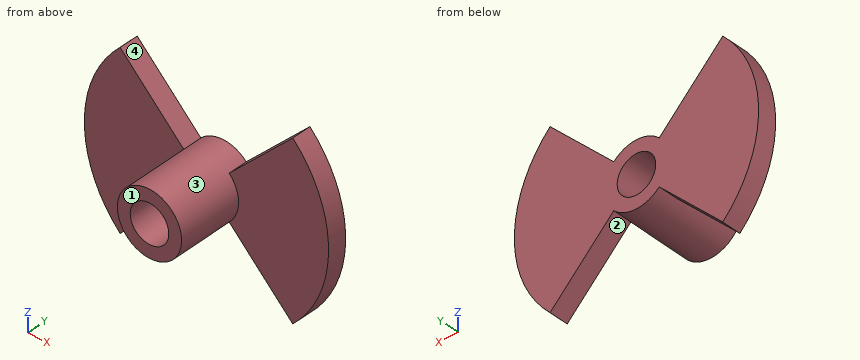
Autodesk Inventor part; units mm, degrees
ref_plane "YZ Plane" through (0, 0, 0) normal (1, 0, 0) x (0, 1, 0)
ref_plane "XZ Plane" through (0, 0, 0) normal (0, 1, 0) x (-1, 0, 0)
ref_plane "XY Plane" through (0, 0, 0) normal (0, 0, 1) x (1, 0, 0)
sketch "Sketch1" plane through (0, 0, 0) normal (0, 1, 0) x (-1, 0, 0)
  circle A0 centre (0, 0) radius 2.5
  circle A1 centre (0, 0) radius 1.5
  dimension "d1" = 3
  dimension "d2" = 1
extrude "Extrusion1" add sketch "Sketch1" along normal blind 5
sketch "Sketch2" plane through (0, 5, 0) normal (0, 1, 0) x (1, 0, 0)
  circle A0 centre (0, 0) radius 1.5
  circle A1 centre (0, 0) radius 9.5
  line L0 (-6.7175, -6.7175) -> (6.7175, 6.7175)
  line L1 (-6.7175, 6.7175) -> (6.7175, -6.7175)
  line L2 (-9.5, 0) -> (9.5, 0) construction
  circle A2 centre (0, 0) radius 2.5
  point P0 (1.7678, -1.7678)
  point P1 (1.7678, 1.7678)
  point P2 (-1.7678, 1.7678)
  point P3 (-1.7678, -1.7678)
  dimension "d5" = 19
  dimension "d6" = 45
  dimension "d7" = 45
extrude "Extrusion2" add sketch "Sketch2" along normal blind 1.5 contours A0 L0 A2 L1 | A0 L1 A2 L0 | L1 A2 L0 A0 | A0 L0 A2 L1 | L0 A1 L1 A2 | A2 L0 A1 L1 picked at (6.8013, -2.1485) picked at (-6.4568, -3.0059)
equation "\"d7\" = d6"
properties part number "Helice"
The listing builds one solid part. Answer for the finished solid, in the listing's coordinates (mm). Face numbers are marked on the shaded views. A direction names the side the tool comes from. Round coordinates to 2 decimals unless told otherwise and drop trailing zeros. Loops run counter-clockwise (first coordinate to the right, second up) from the corner with the lowest first, then second, coordinate; pieces in that order, holes last. Notation, with made-up numbers: (-38, 48) - (-23, 48) arc R6 ccw to (-23, 56) - close; hole circle Ø5 at (2.25, 20). An arc over 180 degrees is marked (long way). Return JSON: item names as keys, results as strings. Group by question number.
1. The part is cut by section C-C on z = -5.25. Determine the outline of the cut face in (x, y).
2. Which of the six approach directions +Z, -Z, +X, -X, +Y, -Y give full straight-line access (tool end or side, diameter ignored) to the marked faces 1, 2, 3 and 4?
3. The part is cut by section B-B on y = 5.75. Determine the outline of the cut face in (x, z).
4. The part is cut by section D-D on z = 2.75. Determine the outline of the cut face in (x, y), then the cut area to 3 significant figures.
5. Each of these flat-tipped pins is pushed along its axis until it touches: P1, Ø3, axis at x = -2.5, z = 5, coming from the +Y side; P2, Ø3, axis at x = 2, y = 3.5, coming from the -Z side; P3, Ø6, axis at x = -7, z = -0.5, coming from the -Y side. Where does it stop, or does it pass through?
6. The part is cut by section A-A on z = -2.25. Determine the outline of the cut face in (x, y).
7. Consider probe 1 along X at (y, z) = (3, 0); probe 2 along Y at (x, z) = (3.25, 2). Determine where each line is inside the solid, lowest interval first.
Resolved:
{
 "1": {"outline": "(-7.92, 5) - (-5.25, 5) - (-5.25, 6.5) - (-7.92, 6.5) - close; (5.25, 5) - (7.92, 5) - (7.92, 6.5) - (5.25, 6.5) - close"},
 "2": {"face 1": "+Z, -Z, +X, -X, -Y", "face 2": "-Z, +Y, -Y", "face 3": "-Y", "face 4": "+Z, +Y, -Y"},
 "3": {"outline": "(-6.72, -6.72) - (-1.77, -1.77) arc R2.5 ccw to (1.77, -1.77) - (6.72, -6.72) arc R9.5 ccw to (6.72, 6.72) - (1.77, 1.77) arc R2.5 ccw to (-1.77, 1.77) - (-6.72, 6.72) arc R9.5 ccw to start; hole circle Ø3 at (0, 0)"},
 "4": {"outline": "(-9.09, 5) - (-2.75, 5) - (-2.75, 6.5) - (-9.09, 6.5) - close; (2.75, 5) - (9.09, 5) - (9.09, 6.5) - (2.75, 6.5) - close", "area": "19.0 mm²"},
 "5": {"P1": "passes through", "P2": "stops at z = -2.45", "P3": "stops at y = 5"},
 "6": {"outline": "(-9.23, 5) - (-2.25, 5) - (-2.25, 6.5) - (-9.23, 6.5) - close; (-1.09, 0) - (1.09, 0) - (1.09, 6.5) - (-1.09, 6.5) - close; (2.25, 5) - (9.23, 5) - (9.23, 6.5) - (2.25, 6.5) - close"},
 "7": {"probe 1": "x = -2.5 to -1.5, 1.5 to 2.5", "probe 2": "y = 5 to 6.5"}
}
